from build123d import *

# Parameters (mm, degrees)
F0_R     = 17.075
F0_R_2   = 16.075
F1_DEPTH = 57
F2_R     = 16.075
F3_DEPTH = 1.4
F4_R     = 16.075
F4_R_2   = 9.7
F5_DEPTH = 1.5


with BuildPart() as f1:
    # F0 (on Top) → F1 (new body)
    with BuildSketch(Plane.XY):
        Circle(F0_R)
        Circle(F0_R_2, mode=Mode.SUBTRACT)
    extrude(amount=-F1_DEPTH)

    # F2 (on face) → F3 (join)
    with BuildSketch(Plane.XY):
        Circle(F2_R)
        with BuildLine():
            ThreePointArc((-10.6883113727, 2.6), (0, 11), (10.6883113727, 2.6))
            Line((10.6883113727, 2.6), (14.7, 2.6))
            Line((14.7, 2.6), (14.7, 0))
            Line((14.7, 0), (14.7, -2.6))
            Line((14.7, -2.6), (10.6883113727, -2.6))
            ThreePointArc((10.6883113727, -2.6), (0, -11), (-10.6883113727, -2.6))
            Line((-10.6883113727, -2.6), (-14.7, -2.6))
            Line((-14.7, -2.6), (-14.7, 0))
            Line((-14.7, 0), (-14.7, 2.6))
            Line((-14.7, 2.6), (-10.6883113727, 2.6))
        make_face(mode=Mode.SUBTRACT)
    extrude(amount=-F3_DEPTH)

    # F4 (on face) → F5 (join)
    with BuildSketch(Plane(origin=(0, 0, -57), x_dir=(1, 0, 0), z_dir=(0, 0, -1))):
        Circle(F4_R)
        Circle(F4_R_2, mode=Mode.SUBTRACT)
    extrude(amount=-F5_DEPTH)


solid = f1.part
Here's how the part is built. I have some questions about the finished solid (model axes, mm). A direction names the side the tool comes from. Round coordinates to 2 decimals unless told otherwise and drop trailing zeros. Order: outer loops, then holes, each group sorted by start corner. A loop starts at its lowest first (then second) coordinate and runs counter-clockwise, first axis right, second up. Notation, with made-up numbers: M 77,-31 L 112,-31 A36 cw 112,7 Z; hole C -6,45 d7. An arc over 180 degrees is marked long. Return JSON: item names as keys, results as strings. Group by question number.
1. Please list where these lines run through material, in increasing order: probe 1 along Y at (x, z) = (0, -29) (3 decimals); probe 2 along Y at (x, z) = (0, -56.45) (3 decimals); probe 3 along Z at (x, y) = (3, 15).
2. If we section it at C-C on z = -33: List the corners of the cut face in (x, y) for me (3 decimals), then the cut area to 3 significant figures.
3. If we mould it in two halves opening along Y, with no side actions, what happens to faces 4 (the face through (-3.7, -16.67, -28.1)), 5 (the face through (9.252, -2.914, -56.26)), 6 (the face through (4, -11, 0)), 7 (the face through (0, -11, -1))? For each: pulls with the +Y half, pulls with the -Y half, needs draft (parallel to the pull), parting line crosses it, or undercut.
4. On a 3-axis mill with a long thin cutter (end or side, diameter ignored), from which of +Z, -Z, +X, -X, +Y, -Y can I reach the whole of each face in a straight line? I mean faces 1 (the face through (7, 7, -57)), 2 (the face through (7, 7, -55.5)), 3 (the face through (13, -2.6, -1)). Say none if no direction works.
5. If we section it at D-D on x = -13.5: List the corners of the cut face in (y, z) for me, then the cut area to 3 significant figures.
6. I'm going to push flat-ended pins straight in: pin 1 Ø5 at (y, z) = (5.5, -34.5) entering from -X; pin 2 Ø1 at (x, z) = (9, -35) entering from +Y; pin 3 Ø8 at (y, z) = (-12.5, -23) entering from -X. Where does each tip first touch, or does it pass through?
7. If we section it at B-B on x = 0: List the corners of the cut face in (y, z) for me (3 decimals), then the cut area to 3 significant figures.
8. If we section it at A-A on y = 0: List the corners of the cut face in (x, z) for me (3 decimals).
Reply:
{
 "1": {"probe 1": "-17.075 to -16.075, 16.075 to 17.075", "probe 2": "-17.075 to -9.7, 9.7 to 17.075", "probe 3": "-57 to -55.5, -1.4 to 0"},
 "2": {"outline": "C 0,0 d34.15; hole C 0,0 d32.15", "area": "104 mm^2"},
 "3": {"face 4": "parting line crosses it", "face 5": "undercut", "face 6": "needs draft", "face 7": "undercut"},
 "4": {"face 1": "-Z, +X, -X, +Y, -Y", "face 2": "none", "face 3": "+Z"},
 "5": {"outline": "M -10.45,-57 L 10.45,-57 L 10.45,0 L 2.6,0 L 2.6,-1.4 L 8.73,-1.4 L 8.73,-55.5 L -8.73,-55.5 L -8.73,-1.4 L -2.6,-1.4 L -2.6,0 L -10.45,0 Z", "area": "240 mm^2"},
 "6": {"pin 1": "x = -16.81", "pin 2": "y = 14.81", "pin 3": "x = -14.81"},
 "7": {"outline": "M -17.075,-57 L -9.7,-57 L -9.7,-55.5 L -16.075,-55.5 L -16.075,-1.4 L -11,-1.4 L -11,0 L -17.075,0 Z; M 9.7,-57 L 17.075,-57 L 17.075,0 L 11,0 L 11,-1.4 L 16.075,-1.4 L 16.075,-55.5 L 9.7,-55.5 Z", "area": "147 mm^2"},
 "8": {"outline": "M -17.075,-57 L -9.7,-57 L -9.7,-55.5 L -16.075,-55.5 L -16.075,-1.4 L -14.7,-1.4 L -14.7,0 L -17.075,0 Z; M 9.7,-57 L 17.075,-57 L 17.075,0 L 14.7,0 L 14.7,-1.4 L 16.075,-1.4 L 16.075,-55.5 L 9.7,-55.5 Z"}
}
